Check sheet for the drawn part. Datum: minimum x, y, z corner. Units: mm. A direction names the side the tool comes from. Coordinates: 2 decimals unless noted, no trailing zeros. Order: outer loops, then holes, each group sorted by start corner. A loop starts at its lowest first (then second) coordinate and runs counter-clockwise, first axis right, second up. Notation, with made-up numbers: (52, -20) - (84, -20) arc R20 cw to (84, 0) - close; hole circle Ø7 at (61.5, 14.25). An arc over 180 degrees is marked (long way). Put each result on its own line as item: value.
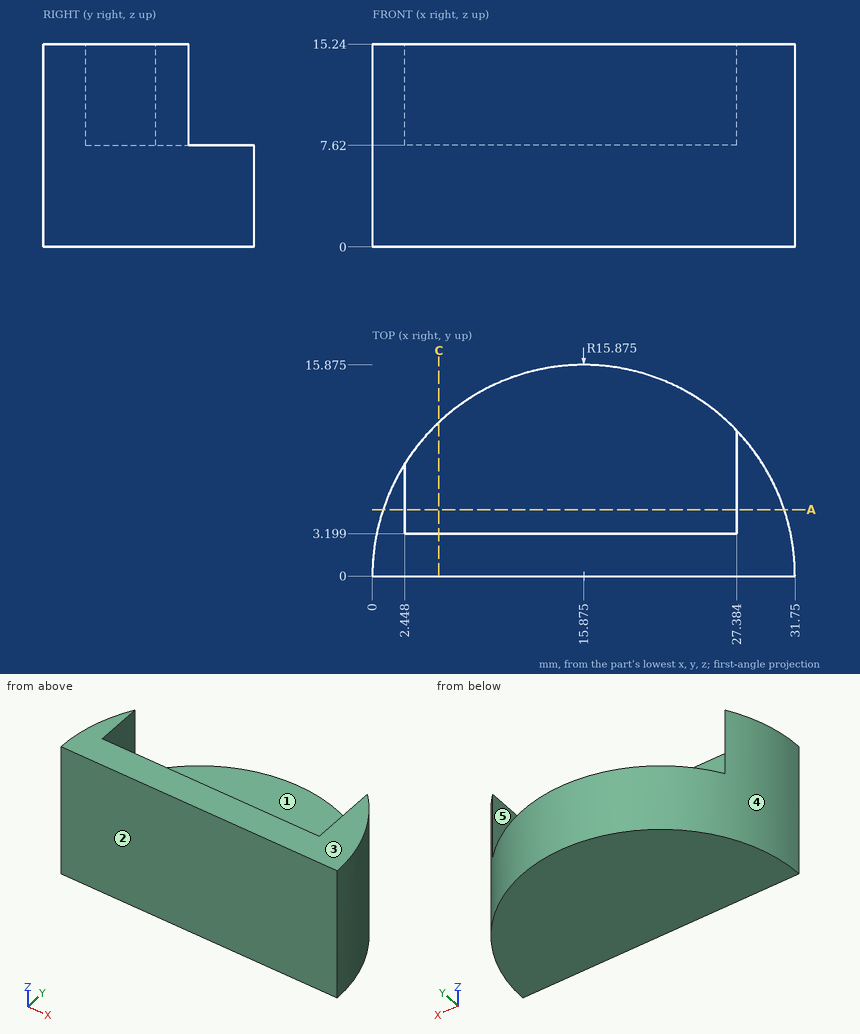
Q1. Thickness scan on L1, parallel to Z at x = 17, y = 12.75; L2, parallel to Y at x = 27, z = 10; L3, parallel to X at y = 0.5, z = 1.25. Record the ranges inside material, lowest first. Write a range as [from, to].
Answer block:
L1: z = [0, 7.62]
L2: y = [0, 3.2]
L3: x = [0.01, 31.74]
Q2. Draft check along X on the marked faces 3, 4 and 5. Enter one of: pulls with the +X half, pulls with the -X half, needs draft (parallel to the pull), parting line crosses it, or undercut.
Answer block:
face 3: needs draft
face 4: parting line crosses it
face 5: undercut
Q3. Section check A-A on y = 5. Record the boundary of the cut face in (x, z), then the cut area to 3 significant figures.
Answer block:
outline: (0.81, 0) - (30.94, 0) - (30.94, 15.24) - (27.38, 15.24) - (27.38, 7.62) - (2.45, 7.62) - (2.45, 15.24) - (0.81, 15.24) - close
area: 269 mm^2
Q4. Access from +Z, -Z, +X, -X, +Y, -Y to the whole of each face (thin tool, end or side, straight path). Record for the marked faces 1 and 2.
Answer block:
face 1: +Z, +Y
face 2: +Z, -Z, +X, -X, -Y
Q5. Depth check by flat-ended pin: pin 1 Ø6 at (x, z) = (18, 2.5) entering from +Y (3 decimals); pin 2 Ø8 at (x, z) = (19.5, 11) entering from +Y (1 decimal); pin 3 Ø4 at (y, z) = (5, 10.5) entering from +X; pin 4 Ø6 at (y, z) = (8.5, 12) entering from -X. Enter the tip coordinate at first touch or a pass-through.
Answer block:
pin 1: stops at y = 15.875
pin 2: stops at y = 15.8
pin 3: stops at x = 31.46
pin 4: stops at x = 0.98
Q6. Section check C-C on x = 5. Record the boundary of the cut face in (y, z) (1 decimal), then the cut area to 4 significant figures.
Answer block:
outline: (0, 0) - (11.6, 0) - (11.6, 7.6) - (3.2, 7.6) - (3.2, 15.2) - (0, 15.2) - close
area: 112.5 mm^2
